Verification items for this drawing (mm, ordinates from the low corner). Coordinates: 2 decimals unless noted, no trailing zeros.
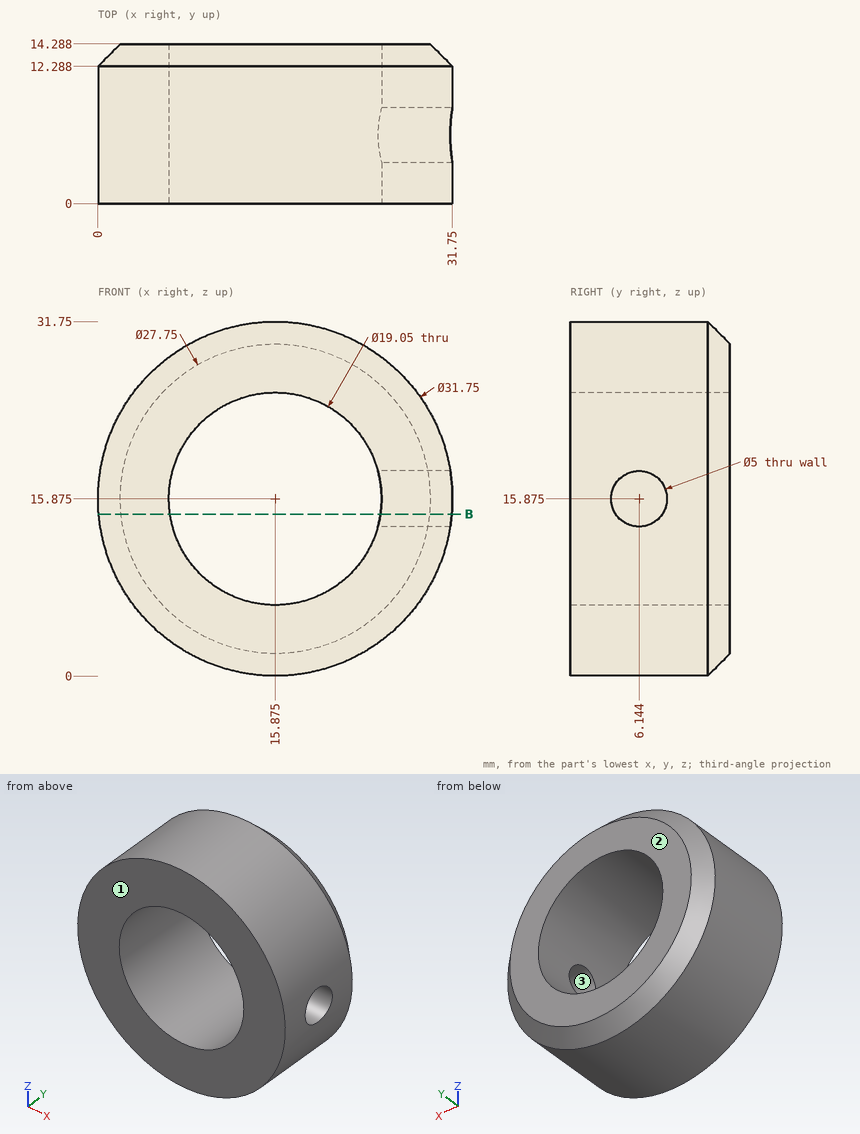
1. Thickness scan on line 1 along Z through (x, y) = (26.5, 8); line 2 along Z through (x, y) = (15, 6) (1 decimal); line 3 along X through (y, z) = (1.25, 20) (1 decimal). Record the ranges inside material, lowest first.
Computed values:
line 1: z = 4.08 to 14.2, 17.55 to 27.67
line 2: z = 0 to 6.4, 25.4 to 31.7
line 3: x = 0.5 to 7.3, 24.5 to 31.2
2. Draft check along Y on the marked faces 1, 2 and 3. Enter one of: released by +Y, released by -Y, zero draft, split by the parting line, or undercut.
Computed values:
face 1: released by -Y
face 2: released by +Y
face 3: undercut
3. Gauge pin test, flat ends, axial feed: pin 1 Ø1.5 at (y, z) = (4, 26) entering from -X (1 decimal); pin 2 Ø2 at (y, z) = (11.5, 3.5) entering from -X; pin 3 Ø5 at (x, z) = (9.5, 15) entering from +Y; pin 4 Ø1.5 at (y, z) = (8, 4) entering from -X. Record the tip position at first contact, or that the pin passes through.
Computed values:
pin 1: stops at x = 3.1
pin 2: stops at x = 4.8
pin 3: passes through
pin 4: stops at x = 4.55
4. Sectioned sample at B-B, the plane z = 14.5. Give the number of separate pieces and of enclosed holes in the cut face, and give its area (3 significant figures).
Computed values:
separate pieces: 3
enclosed holes: 0
area: 152 mm2
